Autodesk Inventor part; units mm, degrees
ref_plane "YZ Plane" through (0, 0, 0) normal (1, 0, 0) x (0, 1, 0)
ref_plane "XZ Plane" through (0, 0, 0) normal (0, 1, 0) x (-1, 0, 0)
ref_plane "XY Plane" through (0, 0, 0) normal (0, 0, 1) x (1, 0, 0)
sketch "Sketch1" plane through (0, 0, 0) normal (0, 0, 1) x (1, 0, 0)
  line L0 (0, -83.185) -> (12.6238, -83.185)
  line L1 (12.6238, -83.185) -> (12.6238, -65.5687)
  arc A0 (12.6238, -61.4313) -> (12.6238, -65.5687) centre (12.7, -63.5) ccw
  line L2 (12.6238, -61.4313) -> (12.6238, -40.1687)
  arc A1 (12.6238, -36.0313) -> (12.6238, -40.1687) centre (12.7, -38.1) ccw
  line L3 (12.6238, -36.0313) -> (12.6238, -14.7687)
  arc A2 (12.6238, -10.6313) -> (12.6238, -14.7687) centre (12.7, -12.7) ccw
  line L4 (12.6238, -10.6313) -> (12.6238, 0)
  line L5 (0, 0) -> (12.6238, 0)
  line L6 (0, 0) -> (0, -83.185)
  line L7 (12.7762, -83.185) -> (25.4, -83.185)
  line L8 (25.4, 0) -> (25.4, -83.185)
  line L9 (12.7762, 0) -> (25.4, 0)
  line L10 (12.7762, -10.6313) -> (12.7762, 0)
  arc A3 (12.7762, -14.7687) -> (12.7762, -10.6313) centre (12.7, -12.7) ccw
  line L11 (12.7762, -36.0313) -> (12.7762, -14.7687)
  arc A4 (12.7762, -40.1687) -> (12.7762, -36.0313) centre (12.7, -38.1) ccw
  line L12 (12.7762, -61.4313) -> (12.7762, -40.1687)
  arc A5 (12.7762, -65.5687) -> (12.7762, -61.4313) centre (12.7, -63.5) ccw
  line L13 (12.7762, -83.185) -> (12.7762, -65.5687)
  line L14 (216.6911, 0) -> (216.6911, 12.6238)
  line L15 (216.6911, 12.6238) -> (206.0725, 12.6238)
  arc A6 (201.9097, 12.6238) -> (206.0725, 12.6238) centre (203.9911, 12.7) ccw
  line L16 (201.9097, 12.6238) -> (180.6725, 12.6238)
  arc A7 (176.5097, 12.6238) -> (180.6725, 12.6238) centre (178.5911, 12.7) ccw
  line L17 (176.5097, 12.6238) -> (155.2725, 12.6238)
  arc A8 (151.1097, 12.6238) -> (155.2725, 12.6238) centre (153.1911, 12.7) ccw
  line L18 (151.1097, 12.6238) -> (129.8725, 12.6238)
  arc A9 (125.7097, 12.6238) -> (129.8725, 12.6238) centre (127.7911, 12.7) ccw
  line L19 (125.7097, 12.6238) -> (104.4725, 12.6238)
  arc A10 (100.3097, 12.6238) -> (104.4725, 12.6238) centre (102.3911, 12.7) ccw
  line L20 (100.3097, 12.6238) -> (79.0725, 12.6238)
  arc A11 (74.9097, 12.6238) -> (79.0725, 12.6238) centre (76.9911, 12.7) ccw
  line L21 (74.9097, 12.6238) -> (53.6725, 12.6238)
  arc A12 (49.5097, 12.6238) -> (53.6725, 12.6238) centre (51.5911, 12.7) ccw
  line L22 (49.5097, 12.6238) -> (28.2725, 12.6238)
  arc A13 (24.1097, 12.6238) -> (28.2725, 12.6238) centre (26.1911, 12.7) ccw
  line L23 (24.1097, 12.6238) -> (2.8725, 12.6238)
  arc A14 (-1.2903, 12.6238) -> (2.8725, 12.6238) centre (0.7911, 12.7) ccw
  line L24 (-1.2903, 12.6238) -> (-22.5275, 12.6238)
  arc A15 (-26.6903, 12.6238) -> (-22.5275, 12.6238) centre (-24.6089, 12.7) ccw
  line L25 (-26.6903, 12.6238) -> (-47.9275, 12.6238)
  arc A16 (-52.0903, 12.6238) -> (-47.9275, 12.6238) centre (-50.0089, 12.7) ccw
  line L26 (-52.0903, 12.6238) -> (-73.3275, 12.6238)
  arc A17 (-77.4903, 12.6238) -> (-73.3275, 12.6238) centre (-75.4089, 12.7) ccw
  line L27 (-77.4903, 12.6238) -> (-98.7275, 12.6238)
  arc A18 (-102.8903, 12.6238) -> (-98.7275, 12.6238) centre (-100.8089, 12.7) ccw
  line L28 (-102.8903, 12.6238) -> (-124.1275, 12.6238)
  arc A19 (-128.2903, 12.6238) -> (-124.1275, 12.6238) centre (-126.2089, 12.7) ccw
  line L29 (-128.2903, 12.6238) -> (-149.5275, 12.6238)
  arc A20 (-153.6903, 12.6238) -> (-149.5275, 12.6238) centre (-151.6089, 12.7) ccw
  line L30 (-153.6903, 12.6238) -> (-174.9275, 12.6238)
  arc A21 (-179.0903, 12.6238) -> (-174.9275, 12.6238) centre (-177.0089, 12.7) ccw
  line L31 (-179.0903, 12.6238) -> (-200.3275, 12.6238)
  arc A22 (-204.4903, 12.6238) -> (-200.3275, 12.6238) centre (-202.4089, 12.7) ccw
  line L32 (-204.4903, 12.6238) -> (-225.7275, 12.6238)
  arc A23 (-229.8903, 12.6238) -> (-225.7275, 12.6238) centre (-227.8089, 12.7) ccw
  line L33 (-229.8903, 12.6238) -> (-251.1275, 12.6238)
  arc A24 (-255.2903, 12.6238) -> (-251.1275, 12.6238) centre (-253.2089, 12.7) ccw
  line L34 (-255.2903, 12.6238) -> (-276.5275, 12.6238)
  arc A25 (-280.6903, 12.6238) -> (-276.5275, 12.6238) centre (-278.6089, 12.7) ccw
  line L35 (-280.6903, 12.6238) -> (-301.9275, 12.6238)
  arc A26 (-306.0903, 12.6238) -> (-301.9275, 12.6238) centre (-304.0089, 12.7) ccw
  line L36 (-306.0903, 12.6238) -> (-327.3275, 12.6238)
  arc A27 (-331.4903, 12.6238) -> (-327.3275, 12.6238) centre (-329.4089, 12.7) ccw
  line L37 (-331.4903, 12.6238) -> (-352.7275, 12.6238)
  arc A28 (-356.8903, 12.6238) -> (-352.7275, 12.6238) centre (-354.8089, 12.7) ccw
  line L38 (-356.8903, 12.6238) -> (-378.1275, 12.6238)
  arc A29 (-382.2903, 12.6238) -> (-378.1275, 12.6238) centre (-380.2089, 12.7) ccw
  line L39 (-382.2903, 12.6238) -> (-403.5275, 12.6238)
  arc A30 (-407.6903, 12.6238) -> (-403.5275, 12.6238) centre (-405.6089, 12.7) ccw
  line L40 (-407.6903, 12.6238) -> (-418.3089, 12.6238)
  line L41 (-418.3089, 12.6238) -> (-418.3089, 0)
  line L42 (-418.3089, 0) -> (216.6911, 0)
  line L43 (216.6911, 12.7762) -> (216.6911, 25.4)
  line L44 (-418.3089, 25.4) -> (216.6911, 25.4)
  line L45 (-418.3089, 25.4) -> (-418.3089, 12.7762)
  line L46 (-418.3089, 12.7762) -> (-407.6903, 12.7762)
  arc A31 (-403.5275, 12.7762) -> (-407.6903, 12.7762) centre (-405.6089, 12.7) ccw
  line L47 (-403.5275, 12.7762) -> (-382.2903, 12.7762)
  arc A32 (-378.1275, 12.7762) -> (-382.2903, 12.7762) centre (-380.2089, 12.7) ccw
  line L48 (-378.1275, 12.7762) -> (-356.8903, 12.7762)
  arc A33 (-352.7275, 12.7762) -> (-356.8903, 12.7762) centre (-354.8089, 12.7) ccw
  line L49 (-352.7275, 12.7762) -> (-331.4903, 12.7762)
  arc A34 (-327.3275, 12.7762) -> (-331.4903, 12.7762) centre (-329.4089, 12.7) ccw
  line L50 (-327.3275, 12.7762) -> (-306.0903, 12.7762)
  arc A35 (-301.9275, 12.7762) -> (-306.0903, 12.7762) centre (-304.0089, 12.7) ccw
  line L51 (-301.9275, 12.7762) -> (-280.6903, 12.7762)
  arc A36 (-276.5275, 12.7762) -> (-280.6903, 12.7762) centre (-278.6089, 12.7) ccw
  line L52 (-276.5275, 12.7762) -> (-255.2903, 12.7762)
  arc A37 (-251.1275, 12.7762) -> (-255.2903, 12.7762) centre (-253.2089, 12.7) ccw
  line L53 (-251.1275, 12.7762) -> (-229.8903, 12.7762)
  arc A38 (-225.7275, 12.7762) -> (-229.8903, 12.7762) centre (-227.8089, 12.7) ccw
  line L54 (-225.7275, 12.7762) -> (-204.4903, 12.7762)
  arc A39 (-200.3275, 12.7762) -> (-204.4903, 12.7762) centre (-202.4089, 12.7) ccw
  line L55 (-200.3275, 12.7762) -> (-179.0903, 12.7762)
  arc A40 (-174.9275, 12.7762) -> (-179.0903, 12.7762) centre (-177.0089, 12.7) ccw
  line L56 (-174.9275, 12.7762) -> (-153.6903, 12.7762)
  arc A41 (-149.5275, 12.7762) -> (-153.6903, 12.7762) centre (-151.6089, 12.7) ccw
  line L57 (-149.5275, 12.7762) -> (-128.2903, 12.7762)
  arc A42 (-124.1275, 12.7762) -> (-128.2903, 12.7762) centre (-126.2089, 12.7) ccw
  line L58 (-124.1275, 12.7762) -> (-102.8903, 12.7762)
  arc A43 (-98.7275, 12.7762) -> (-102.8903, 12.7762) centre (-100.8089, 12.7) ccw
  line L59 (-98.7275, 12.7762) -> (-77.4903, 12.7762)
  arc A44 (-73.3275, 12.7762) -> (-77.4903, 12.7762) centre (-75.4089, 12.7) ccw
  line L60 (-73.3275, 12.7762) -> (-52.0903, 12.7762)
  arc A45 (-47.9275, 12.7762) -> (-52.0903, 12.7762) centre (-50.0089, 12.7) ccw
  line L61 (-47.9275, 12.7762) -> (-26.6903, 12.7762)
  arc A46 (-22.5275, 12.7762) -> (-26.6903, 12.7762) centre (-24.6089, 12.7) ccw
  line L62 (-22.5275, 12.7762) -> (-1.2903, 12.7762)
  arc A47 (2.8725, 12.7762) -> (-1.2903, 12.7762) centre (0.7911, 12.7) ccw
  line L63 (2.8725, 12.7762) -> (24.1097, 12.7762)
  arc A48 (28.2725, 12.7762) -> (24.1097, 12.7762) centre (26.1911, 12.7) ccw
  line L64 (28.2725, 12.7762) -> (49.5097, 12.7762)
  arc A49 (53.6725, 12.7762) -> (49.5097, 12.7762) centre (51.5911, 12.7) ccw
  line L65 (53.6725, 12.7762) -> (74.9097, 12.7762)
  arc A50 (79.0725, 12.7762) -> (74.9097, 12.7762) centre (76.9911, 12.7) ccw
  line L66 (79.0725, 12.7762) -> (100.3097, 12.7762)
  arc A51 (104.4725, 12.7762) -> (100.3097, 12.7762) centre (102.3911, 12.7) ccw
  line L67 (104.4725, 12.7762) -> (125.7097, 12.7762)
  arc A52 (129.8725, 12.7762) -> (125.7097, 12.7762) centre (127.7911, 12.7) ccw
  line L68 (129.8725, 12.7762) -> (151.1097, 12.7762)
  arc A53 (155.2725, 12.7762) -> (151.1097, 12.7762) centre (153.1911, 12.7) ccw
  line L69 (155.2725, 12.7762) -> (176.5097, 12.7762)
  arc A54 (180.6725, 12.7762) -> (176.5097, 12.7762) centre (178.5911, 12.7) ccw
  line L70 (180.6725, 12.7762) -> (201.9097, 12.7762)
  arc A55 (206.0725, 12.7762) -> (201.9097, 12.7762) centre (203.9911, 12.7) ccw
  line L71 (206.0725, 12.7762) -> (216.6911, 12.7762)
  line L72 (-37.3089, 25.4) -> (64.2911, 25.4)
  line L73 (64.2911, 25.4) -> (64.2911, 0)
  line L74 (64.2911, 0) -> (-37.3089, 0)
  line L75 (-37.3089, 0) -> (-37.3089, 25.4)
  line L76 (0, 0) -> (25.4, 0)
  line L77 (25.4, 0) -> (25.4, -83.185)
  line L78 (25.4, -83.185) -> (0, -83.185)
  line L79 (0, -83.185) -> (0, 0)
  circle A56 centre (-24.6089, 12.7) radius 2.0828
  circle A57 centre (0.7911, 12.7) radius 2.0828
  circle A58 centre (26.1911, 12.7) radius 2.0828
  circle A59 centre (51.5911, 12.6238) radius 2.0267
  circle A60 centre (12.7, -12.7) radius 2.0701
  circle A61 centre (12.7, -38.1) radius 2.0701
  circle A62 centre (12.7, -63.5) radius 2.0701
  line L80 (242.0911, -84.7725) -> (-443.7089, -84.7725)
  line L81 (242.0911, -84.7725) -> (-443.7089, -84.7725)
  line L82 (-443.7089, -86.36) -> (-443.7089, -84.7725)
  line L83 (-442.1214, -86.36) -> (-443.7089, -86.36)
  line L84 (-442.1214, -86.36) -> (240.5036, -86.36)
  line L85 (242.0911, -86.36) -> (240.5036, -86.36)
  line L86 (242.0911, -84.7725) -> (242.0911, -86.36)
  line L87 (-442.1214, -137.16) -> (-442.1214, -86.36)
  line L88 (-442.1214, -137.16) -> (240.5036, -137.16)
  line L89 (240.5036, -86.36) -> (240.5036, -137.16)
  line L90 (-442.1214, -86.36) -> (240.5036, -86.36)
  line L91 (0, -83.185) -> (25.4, -83.185)
  line L92 (0, -83.185) -> (25.4, -83.185)
  line L93 (25.4, -84.7725) -> (0, -84.7725)
  line L94 (-5.08, -83.185) -> (30.48, -83.185)
  line L95 (-5.08, -83.185) -> (30.48, -83.185)
  line L96 (-5.08, -83.185) -> (30.48, -83.185)
extrude "Plate1" add sketch "Sketch1" along normal blind 3.175 contours L6 L5 L4 A2 L3 A1 L2 A0 L1 L0 | L1 A62 L13 L78 | L42 L75 L25 A15 L24 A14 L23 A13 L22 A12 A59 L21 L73 L9 L5 | L13 A5 L12 A4 L11 A3 L10 L9 L8 L7 | L42 L10 A60 L4 | L2 A61 L12 A62 | L75 L61 A56 L25 | A60 L11 A61 L3 | L75 L44 L73 L65 A49 L64 A48 L63 A47 L62 A46 L61 | A56 L62 A57 L24 | L21 A12 A59 L22 A58 L64 A49 L65 L73 | A57 L63 A58 L23
sketch "Sketch4" plane through (25.4, -83.185, 3.175) normal (0, -1, 0) x (1, 0, 0)
  line L0 (-25.4, 0) -> (0, 0)
  line L1 (0, 0) -> (0, 85.725)
  line L2 (0, 85.725) -> (-25.4, 85.725)
  line L3 (-25.4, 85.725) -> (-25.4, 0)
edge flange "Flange2" height 88.9 angle 90 thickness 3.175 bend radius 1.27 thickness toward (0, -1, 0) relief tear relief width 3.175 relief depth 1.5875 edges at (12.7, -83.185, 3.175) wall of the first edge with corners at (0, -83.185, 3.175) (25.4, -83.185, 3.175) (25.4, -83.185, 88.9) (0, -83.185, 88.9)
bend "Bend2"
corner "Corner2"
sketch "Sketch5" plane through (0, -83.185, 88.9) normal (0, 1, 0) x (1, 0, 0)
  line L0 (0, 84.455) -> (25.4, 0)
  line L1 (0, 0) -> (25.4, 84.455)
  circle A0 centre (12.7, 42.2275) radius 3.3782
  point P0 (0, 88.9)
  dimension "d29" = 6.7564
hole "Hole2" at (12.7, -83.185, 46.6725) direction (0, -1, 0) diameter 6.7564 end through all
equation "\"d35\" = Thickness"
equation "\"d19\" = BendReliefWidth"
equation "\"d20\" = BendReliefDepth"
equation "\"d21\" = MinimumRemnant"
equation "\"d22\" = BendRadius"
equation "\"d26\" = CornerReliefSize"
equation "\"d27\" = GapSize"
equation "\"d28\" = JacobiRadiusSize"
equation "\"BendRadius\" = Thickness"
equation "\"BendReliefWidth\" = Thickness"
equation "\"BendReliefDepth\" = 0.5 * Thickness"
equation "\"CornerReliefSize\" = 4 * Thickness"
equation "\"MinimumRemnant\" = 2 * Thickness"
equation "\"TransitionRadius\" = BendRadius"
equation "\"JacobiRadiusSize\" = BendRadius"
equation "\"GapSize\" = Thickness"
equation "\"d0\" = BendRadius"
properties part number "Angle attach bracket"
Could you check a few things on this model? Use its own coordinates, in mm. A direction names the side the tool comes from. Give positions to 0.01 mm unless a question says otherwise; leave off trailing zeros. Write each loop counter-clockwise with the first axis right and the second up, starting at its lowest first coordinate (ties: lowest second). Pieces come first, ordered by that corner, then holes. Notation, with made-up numbers: (66, -25.5) -> (107, -25.5) arc R12 cw to (107, -4.5) -> close; hole circle Ø4 at (29, 5). An arc over 180 degrees is marked (long way). Write each question's results on one line, items separated by ' | '.
1. I want a section at D-D, the plane y = 2. Write out the boundary of the cut face in (x, z) (3 decimals).
Check sheet entries:
outline: (-37.309, 0) -> (64.291, 0) -> (64.291, 3.175) -> (-37.309, 3.175) -> close
2. Will these pins go through, and if not, where does the flat tip stop? pin 1 Ø1 at (x, z) = (-27.5, 1) entering from -Y; pin 2 Ø20.5 at (x, z) = (7, 32.5) entering from +Y (3 decimals); pin 3 Ø4 at (x, z) = (12.7, 46.67) entering from -Y; pin 4 Ø4.5 at (x, y) = (51.59, 12.62) entering from +Z (3 decimals).
Check sheet entries:
pin 1: stops at y = 0 | pin 2: stops at y = -83.185 | pin 3: passes through | pin 4: stops at z = 3.175
3. I want a section at B-B, the plane x = 19.5. Write out the boundary of the cut face in (y, z) (3 decimals), then the cut area to 3 significant figures.
Check sheet entries:
outline: (-86.36, 4.445) arc R4.445 ccw to (-81.915, 0) -> (25.4, 0) -> (25.4, 3.175) -> (-81.915, 3.175) arc R1.27 cw to (-83.185, 4.445) -> (-83.185, 88.9) -> (-86.36, 88.9) -> close | area: 623 mm²
4. I want a section at A-A, the plane y = -38.1. Write out the boundary of the cut face in (x, z) (3 decimals).
Check sheet entries:
outline: (0, 0) -> (10.63, 0) -> (10.63, 3.175) -> (0, 3.175) -> close; (14.77, 0) -> (25.4, 0) -> (25.4, 3.175) -> (14.77, 3.175) -> close
5. I need wall thicknesses on L1, parallel to Z at x = 1, y = -17 (3 decimals); L2, parallel to Y at x = 5, z = 36.5 (3 decimals); L3, parallel to Z at x = 12, y = -84. Which ranges of each line are inside material? Lowest first, please.
Check sheet entries:
L1: z = 0 to 3.175 | L2: y = -86.36 to -83.185 | L3: z = 0.52 to 43.37, 49.98 to 88.9
6. I want a section at C-C, the plane z = 25. Write out the boundary of the cut face in (x, y) (3 decimals), then the cut area to 3 significant figures.
Check sheet entries:
outline: (0, -86.36) -> (25.4, -86.36) -> (25.4, -83.185) -> (0, -83.185) -> close | area: 80.6 mm²
7. On a 3-axis mill with a long thin cutter (end or side, diameter ignored), from which of +Z, -Z, +X, -X, +Y, -Y can I reach the whole of each face in a straight line? I mean faces 1 (the flat face through (7, -83.185, 46)), 2 (the flat face through (45, 0, 2)), 3 (the flat face through (0, -85, 25)). Say none if no direction works.
Check sheet entries:
face 1: +Z, +X, -X, +Y | face 2: +Z, -Z, +X, -Y | face 3: +Z, -Z, -X, -Y
8. If we mould it in two halves opening along Z, with no side actions, what happens to faces 4 (the flat face through (13, -16, 3.175)), 5 (the cylindrical face through (12.551, -84.795, 43.298)), 6 (the flat face through (7, -86.36, 47))? For each: released by +Z, released by -Z, zero draft, split by the parting line, or undercut.
Check sheet entries:
face 4: released by +Z | face 5: undercut | face 6: zero draft
